Autodesk Fusion 360 part; units mm, degrees
sketch "Sketch1" plane through (0, 0, 0) normal (0, 0, 1) x (1, 0, 0)
  line L0 (0, 0) -> (2, 0)
  line L1 (2, 0) -> (2, -3)
  line L2 (2, -3) -> (0, -3)
  line L3 (0, -3) -> (0, 0)
  dimension "d8" = 2
  dimension "d9" = 3
extrude "Extrude1" add sketch "Sketch1" along normal blind 60
sketch "Sketch2" plane through (0, -3, 0) normal (0, -1, 0) x (1, 0, 0)
  line L0 (0, 0) -> (2, 0)
  line L1 (2, 0) -> (2, 60)
  line L2 (2, 60) -> (0, 60)
  line L3 (0, 60) -> (0, 0)
  line L4 (0.1, 3) -> (1.9, 3)
  line L5 (1.9, 3) -> (1.9, 5)
  line L6 (1.9, 5) -> (0.1, 5)
  line L7 (0.1, 5) -> (0.1, 3)
  dimension "d12" = 1.8
  dimension "d13" = 2
  dimension "d16" = 3
  dimension "d17" = 0.1
extrude "Extrude2" add sketch "Sketch2" along normal blind 5 contours L4 L5 L6 L7
equation "length = 60 mm"
equation "width = 3 mm"
equation "height = 2 mm"
equation "dent_length = 5 mm"
equation "dent_width = 2 mm"
equation "dent_height = 1.8 mm"
equation "dent_distance = 3 mm"
equation "d8 = height"
equation "d9 = width"
equation "d10 = length"
equation "d12 = dent_height"
equation "d13 = dent_width"
equation "d14 = dent_length"
equation "d16 = dent_distance"
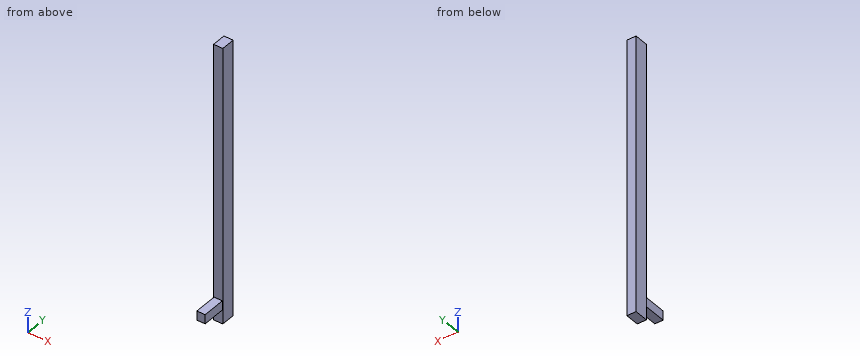
Geometry check sheet. Reference: the model listing, model coordinates, mm. Coordinates: 2 decimals unless noted, no trailing zeros. Order: outer loops, then holes, each group sorted by start corner. A loop starts at its lowest first (then second) coordinate and runs counter-clockwise, first axis right, second up. Notation, with made-up numbers: (84, -20.5) - (139, -20.5) arc R16 cw to (139, -7.5) - close; hole circle Ø3 at (-29, 42.5). An arc over 180 degrees is marked (long way). Answer in a Markdown table with one row per item. Add a question column.
1) Gauge pin test, flat ends, axial feed: P1, Ø1, axis at y = -6.5, z = 4, coming from the -X side; P2, Ø0.5, axis at x = 1, y = -5, coming from the -Z side; P3, Ø2, axis at y = -6.5, z = 4.5, coming from the +X side. Record the tip position at first contact, or that the pin passes through.
2) Cross-section at D-D, the plane z = 26. Record the cut outline in (x, y), then the cut area to 3 significant figures.
3) Cross-section at A-A, the plane z = 4. Record the cut outline in (x, y), then the cut area to 3 significant figures.
4) Cross-section at C-C, the plane y = -4.75. Record the cut outline in (x, z), then the cut area to 3 significant figures.
5) Material ranges on line 1 along Z through (x, y) = (0.9, -3.5); line 2 along Y through (x, z) = (1.45, 45.5), recorded low to high. Write a range as [from, to].
6) Cross-section at B-B, the plane x = 1. Record the cut outline in (y, z).
Check result:
| question | item | result |
|---|---|---|
| 1 | P1 | stops at x = 0.1 |
| 1 | P2 | stops at z = 3 |
| 1 | P3 | stops at x = 1.9 |
| 2 | outline | (0, -3) - (2, -3) - (2, 0) - (0, 0) - close |
| 2 | area | 6.00 mm² |
| 3 | outline | (0, -3) - (0.1, -3) - (0.1, -8) - (1.9, -8) - (1.9, -3) - (2, -3) - (2, 0) - (0, 0) - close |
| 3 | area | 15.0 mm² |
| 4 | outline | (0.1, 3) - (1.9, 3) - (1.9, 5) - (0.1, 5) - close |
| 4 | area | 3.60 mm² |
| 5 | line 1 | z = [3, 5] |
| 5 | line 2 | y = [-3, 0] |
| 6 | outline | (-8, 3) - (-3, 3) - (-3, 0) - (0, 0) - (0, 60) - (-3, 60) - (-3, 5) - (-8, 5) - close |
